Build history of the part. All positions in model axes, mm. Face numbers are marked on the shaded views. A direction names the side the tool comes from. Coordinates: 2 decimals unless noted, no trailing zeros. Loops run counter-clockwise (first coordinate to the right, second up) from the corner with the lowest first, then second, coordinate; pieces in that order, holes last.
(1) Tool access for the marked faces 1 and 2: list every direction of +Z, -Z, +X, -X, +Y, -Y with a clear straight run to the whole face (end or side of a thin tool).
(2) Slice it at C-C (y = 116). Give the cut face in (x, z).
(3) Slice it at D-D (x = -0.5). Give the cut face in (y, z).
(4) Slice it at A-A (x = 13). Give the cut face in (y, z), and give its area (3 significant figures).
(5) Wall check: L1, parallel to X at y = 167, z = 4.5; L2, parallel to Y at x = -11, z = 4.5; L3, parallel to X at y = 122, z = 0.25. Give the ranges that are in metal, low to high.
(6) Flat gauge pins, fed straight in: P1, Ø5, axis at y = 43, z = 0.5, coming from the +X side; P2, Ø5.5, axis at y = 2.5, z = 0.5, coming from the -X side; P3, Ø5, axis at x = -22, z = 2.5, coming from the +Y side. Where does each tip first touch, or does it go through?
(7) Slice it at B-B (z = 0). Give the cut face in (x, y), and give its area (3 significant figures).
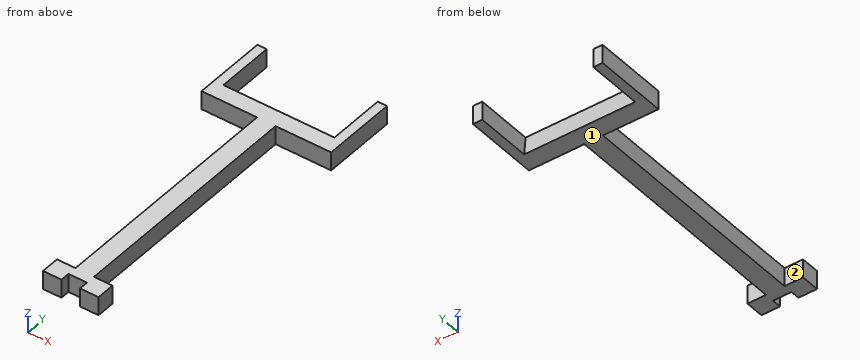
Autodesk Inventor part; units mm, degrees
ref_plane "Work Plane1" through (0, 150, 5) normal (1, 0, 0) x (0, 0, -1)
ref_plane "YZ Plane" through (0, 0, 0) normal (1, 0, 0) x (0, 1, 0)
ref_plane "XZ Plane" through (0, 0, 0) normal (0, 1, 0) x (-1, 0, 0)
sketch "Sketch2" plane through (0, 0, 0) normal (0, 0, 1) x (1, 0, 0)
  line L0 (0, 0) -> (0, 50) construction
  line L1 (0, 0) -> (0, 5)
  line L2 (0, 5) -> (-5, 5)
  line L3 (-5, 5) -> (-5, 0)
  line L4 (-5, 0) -> (-15, 0)
  line L5 (-15, 0) -> (-15, 5)
  line L6 (-15, 5) -> (-15, 10)
  line L7 (-15, 10) -> (-5, 10)
  line L8 (-5, 10) -> (-5, 140)
  line L9 (-5, 140) -> (-35, 140)
  line L10 (-35, 140) -> (-35, 180)
  line L11 (-35, 180) -> (-30, 180)
  line L12 (-30, 180) -> (-30, 150)
  line L13 (-30, 150) -> (0, 150)
  line L14 (0, 5) -> (5, 5)
  line L15 (5, 5) -> (5, 0)
  line L16 (15, 0) -> (15, 5)
  line L17 (15, 5) -> (15, 10)
  line L18 (15, 10) -> (5, 10)
  line L19 (5, 10) -> (5, 140)
  line L20 (5, 140) -> (35, 140)
  line L21 (35, 140) -> (35, 180)
  line L22 (35, 180) -> (30, 180)
  line L23 (30, 180) -> (30, 150)
  line L24 (30, 150) -> (0, 150)
  line L25 (5, 0) -> (15, 0)
  dimension "d6" = 50
  dimension "d7" = 5
  dimension "d8" = 5
  dimension "d9" = 10
  dimension "d10" = 130
  dimension "d11" = 30
  dimension "d12" = 40
  dimension "d13" = 5
  dimension "d14" = 30
  dimension "d21" = 5
  dimension "d22" = 5
  dimension "d24" = 0
extrude "Extrusion1" add sketch "Sketch2" along normal mid plane 10
ref_plane "Work Plane1" through (0, 150, 5) normal (1, 0, 0) x (0, 0, -1)
sketch "Sketch3" plane through (0, 150, 5) normal (1, 0, 0) x (0, 0, -1)
  line L0 (0, 0) -> (10, 0)
  line L1 (0, 0) -> (0, -1)
  line L2 (10, -10) -> (0, -10)
  line L3 (0, -1) -> (10, 0)
  point P0 (5, -150)
  dimension "d27" = 1
extrude "Extrusion2" cut sketch "Sketch3" along normal mid plane 60
properties part number "Sorting Holder x1"
Response values:
1. face 1: -Z, +X, -X, +Y, -Y
1. face 2: +Z, -Z, -X
2. outline: (-5, -5) - (5, -5) - (5, 5) - (-5, 5) - close
3. outline: (5, -5) - (150, -5) - (149, 5) - (5, 5) - close
4. outline: (0, -5) - (10, -5) - (10, 5) - (0, 5) - close; (140, -5) - (150, -5) - (149, 5) - (140, 5) - close
4. area: 195 mm2
5. L1: x = -35 to -30, 30 to 35
5. L2: y = 0 to 10, 140 to 149.05
5. L3: x = -5 to 5
6. P1: stops at x = 5
6. P2: stops at x = -15
6. P3: stops at y = 149.5
7. outline: (-35, 140) - (-5, 140) - (-5, 10) - (-15, 10) - (-15, 0) - (-5, 0) - (-5, 5) - (5, 5) - (5, 0) - (15, 0) - (15, 10) - (5, 10) - (5, 140) - (35, 140) - (35, 180) - (30, 180) - (30, 149.5) - (-30, 149.5) - (-30, 180) - (-35, 180) - close
7. area: 2,520 mm2
